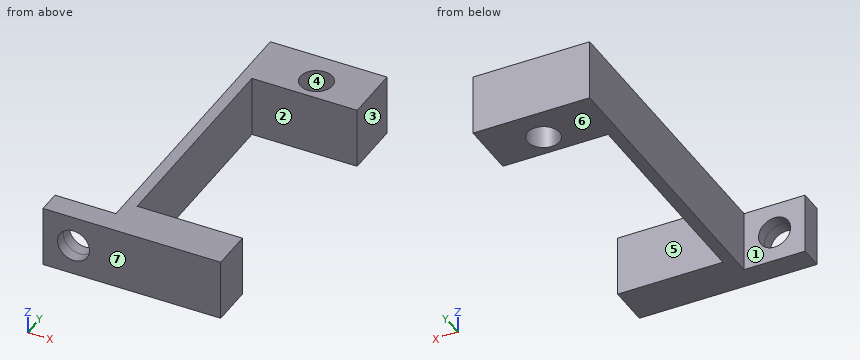
```python
from build123d import *
from build123d.topology import SkipClean

# Parameters (mm, degrees)
SKETCH1_W            = 8
SKETCH1_H            = 8
SKETCH1_R            = 2.1
BOSS_EXTRUDE6_DEPTH  = 1.5
SKETCH6_W            = 8
SKETCH6_H            = 1.5
BOSS_EXTRUDE7_DEPTH  = 15.3
BOSS_EXTRUDE8_START  = 1.5
SKETCH10_W           = 8
SKETCH10_H           = 8
SKETCH10_R           = 2.1
BOSS_EXTRUDE8_DEPTH  = 1.5
SKETCH11_W           = 1.5
SKETCH11_H           = 8
BOSS_EXTRUDE9_DEPTH  = 40.3
SKETCH12_W           = 8
SKETCH12_H           = 7.5
BOSS_EXTRUDE10_DEPTH = 13.8
SKETCH14_R           = 2.1
CUT_EXTRUDE1_DEPTH   = 13.8
SKETCH15_W           = 13.8
SKETCH15_H           = 8
BOSS_EXTRUDE11_DEPTH = 3.95


with BuildPart() as part:
    # Sketch1 → Boss-Extrude6 (new body)
    with BuildSketch(Plane(origin=(0, 0, 0), x_dir=(1, 0, 0), z_dir=(0, 1, 0))):
        with Locations((-4, -4)):
            Rectangle(SKETCH1_W, SKETCH1_H)
        with Locations(Location((-4, -4, 0), (0, 0, 270))):
            Circle(SKETCH1_R, mode=Mode.SUBTRACT)
    extrude(amount=BOSS_EXTRUDE6_DEPTH)



with BuildPart() as body_2:
    # Sketch6 → Boss-Extrude7 (new body)
    with BuildSketch(Plane(origin=(0, 0, 0), x_dir=(0, 0, -1), z_dir=(1, 0, 0))):
        with Locations((-4, -0.75)):
            Rectangle(SKETCH6_W, SKETCH6_H)
    extrude(amount=BOSS_EXTRUDE7_DEPTH)


with BuildPart() as part_1:
    with SkipClean():  # the faces are left unmerged after this step: merging them gives an invalid solid
        add(part.part)

        add(body_2.part)  # Boss-Extrude8 merges body 2
        # Sketch10 → Boss-Extrude8 (add)
        with BuildSketch(Plane.XZ.offset(BOSS_EXTRUDE8_START)):
            with Locations((-4, 4)):
                Rectangle(SKETCH10_W, SKETCH10_H)
            with Locations(Location((-4, 4, 0), (0, 0, 270))):
                Circle(SKETCH10_R, mode=Mode.SUBTRACT)
        extrude(amount=-BOSS_EXTRUDE8_DEPTH)

    # Sketch11 → Boss-Extrude9 (add)
    with SkipClean():  # the faces are left unmerged after this step: merging them gives an invalid solid
        with BuildSketch(Plane(origin=(0, 0, 0), x_dir=(1, 0, 0), z_dir=(0, 1, 0))):
            with Locations((0.75, -4)):
                Rectangle(SKETCH11_W, SKETCH11_H)
        extrude(amount=BOSS_EXTRUDE9_DEPTH)

    # Sketch12 → Boss-Extrude10 (add)
    with SkipClean():  # the faces are left unmerged after this step: merging them gives an invalid solid
        with BuildSketch(Plane(origin=(1.5, 0, 0), x_dir=(0, 0, -1), z_dir=(1, 0, 0))):
            with Locations((-4, 36.55)):
                Rectangle(SKETCH12_W, SKETCH12_H)
        extrude(amount=BOSS_EXTRUDE10_DEPTH)

    # Sketch14 → Cut-Extrude1 (cut)
    with SkipClean():  # the faces are left unmerged after this step: merging them gives an invalid solid
        with BuildSketch(Plane.XY.offset(8)):
            with Locations((8.4, 35.8)):
                Circle(SKETCH14_R)
        extrude(amount=-CUT_EXTRUDE1_DEPTH, mode=Mode.SUBTRACT)

    # Sketch15 → Boss-Extrude11 (add)
    with SkipClean():  # the faces are left unmerged after this step: merging them gives an invalid solid
        with BuildSketch(Plane(origin=(0, 0, 0), x_dir=(1, 0, 0), z_dir=(0, 1, 0))):
            with Locations((8.4, -4)):
                Rectangle(SKETCH15_W, SKETCH15_H)
        extrude(amount=BOSS_EXTRUDE11_DEPTH)


solid = part_1.part
```
Input: part model. Units: mm. Frame: model coordinates. Face numbers are marked on the shaded views. A direction names the side the tool comes from. Give positions to 0.01 mm unless a question says otherwise; leave off trailing zeros. Loops run counter-clockwise (first coordinate to the right, second up) from the corner with the lowest first, then second, coordinate; pieces in that order, holes last. Notation, with made-up numbers: (-34, 42) -> (-9, 42) arc R29 ccw to (-9, 68) -> close; hole circle Ø4 at (-16.75, 18.25). An arc over 180 degrees is marked (long way). Use a Markdown table: item, result.
Q1. Section query C-C, the plane x = 13.75. Return the cut outline in (y, z).
Entries:
| item | result |
|---|---|
| outline | (-1.5, 0) -> (3.95, 0) -> (3.95, 8) -> (-1.5, 8) -> close; (32.8, 0) -> (40.3, 0) -> (40.3, 8) -> (32.8, 8) -> close |
Q2. Pull-direction query (Y, two-part tool) for the marked faces 4, 5, 6 and 7; classes: pulls with the +Y half, pulls with the -Y half, needs draft (parallel to the pull), parting line crosses it, or undercut.
Entries:
| item | result |
|---|---|
| face 4 | undercut |
| face 5 | undercut |
| face 6 | needs draft |
| face 7 | pulls with the -Y half |
Q3. Ray query, probe 1 along Y at (x, z) = (8.4, 4.75); probe 2 along Y at (x, z) = (13, 1.5); probe 3 along Z at (x, y) = (-4, -0.8). Return the intervals inside material, ascending. Write a range as from..to.
Entries:
| item | result |
|---|---|
| probe 1 | y = -1.5..3.95, 32.8..33.7, 37.9..40.3 |
| probe 2 | y = -1.5..3.95, 32.8..40.3 |
| probe 3 | z = 0..1.9, 6.1..8 |
Q4. Section query D-D, the plane z = 6.75. Return the cut outline in (x, y).
Entries:
| item | result |
|---|---|
| outline | (-8, -1.5) -> (15.3, -1.5) -> (15.3, 3.95) -> (1.5, 3.95) -> (1.5, 32.8) -> (15.3, 32.8) -> (15.3, 40.3) -> (0, 40.3) -> (0, 1.5) -> (-8, 1.5) -> close; hole circle Ø4.2 at (8.4, 35.8) |
Q5. Section query B-B, the plane y = 35.8. Return the cut outline in (x, z), plus the area to 3 significant figures.
Entries:
| item | result |
|---|---|
| outline | (0, 0) -> (6.3, 0) -> (6.3, 8) -> (0, 8) -> close; (10.5, 0) -> (15.3, 0) -> (15.3, 8) -> (10.5, 8) -> close |
| area | 88.8 mm² |
Q6. Access query for the marked faces 1, 2 and 3. Directions: +Z, -Z, +X, -X, +Y, -Y. A direction counts if a zero-diameter tool reaches every point of the face in a straight line with its end or side. Return the directions, or none.
Entries:
| item | result |
|---|---|
| face 1 | +Z, -Z, -X, +Y |
| face 2 | +Z, -Z, +X |
| face 3 | +Z, -Z, +X, +Y, -Y |
Q7. Section query A-A, the plane z = 4. Return the cut outline in (x, y), plus the area to 3 significant figures.
Entries:
| item | result |
|---|---|
| outline | (-8, -1.5) -> (-6.1, -1.5) -> (-6.1, 1.5) -> (-8, 1.5) -> close; (-1.9, -1.5) -> (15.3, -1.5) -> (15.3, 3.95) -> (1.5, 3.95) -> (1.5, 32.8) -> (15.3, 32.8) -> (15.3, 40.3) -> (0, 40.3) -> (0, 1.5) -> (-1.9, 1.5) -> close; hole circle Ø4.2 at (8.4, 35.8) |
| area | 239 mm² |
Q8. First-contact query: P1, Ø4, axis at y = 16.5, z = 3, coming from the -X side; P2, Ø2, axis at x = 12.5, y = 32, coming from the -Z side; P3, Ø4, axis at y = 14, z = 2.5, coming from the +X side. Flat tips, straight axial feed; report the tip coordinate or a pass-through.
Entries:
| item | result |
|---|---|
| P1 | stops at x = 0 |
| P2 | stops at z = 0 |
| P3 | stops at x = 1.5 |
